Autodesk Inventor part; units mm, degrees
ref_plane "YZ Plane" through (0, 0, 0) normal (1, 0, 0) x (0, 1, 0)
ref_plane "XZ Plane" through (0, 0, 0) normal (0, 1, 0) x (-1, 0, 0)
ref_plane "XY Plane" through (0, 0, 0) normal (0, 0, 1) x (1, 0, 0)
sketch "Sketch1" plane through (0, 0, 0) normal (0, 0, 1) x (1, 0, 0)
  line L0 (10.3923, 0) -> (5.1962, -9)
  line L1 (5.1962, -9) -> (-5.1962, -9)
  line L2 (-5.1962, -9) -> (-10.3923, 0)
  line L3 (-10.3923, 0) -> (-5.1962, 9)
  line L4 (-5.1962, 9) -> (5.1962, 9)
  line L5 (5.1962, 9) -> (10.3923, 0)
  point P0 (0, 0)
  point P1 (0, 0)
  dimension "d0" = 18
extrude "Extrusion1" add sketch "Sketch1" along normal blind 2.8
sketch "Sketch2" plane through (0, 0, 2.8) normal (0, 0, 1) x (1, 0, 0)
  circle A0 centre (0, 0) radius 6
  dimension "d3" = 12
extrude "Extrusion2" cut sketch "Sketch2" against normal through all
chamfer "Chamfer1" distance 1 angle 45 6 edges at (5.1962, 9, 1.4) (-5.1962, 9, 1.4) (10.3923, 0, 1.4) (5.1962, -9, 1.4) (-5.1962, -9, 1.4) (-10.3923, 0, 1.4)
chamfer "Chamfer2" distance 0.5 angle 45 12 edges at (-9.8923, 0, 2.8) (-4.9462, -8.567, 2.8) (4.9462, -8.567, 2.8) (9.8923, 0, 2.8) (4.9462, 8.567, 2.8) (-4.9462, 8.567, 2.8) (-4.9462, 8.567, 0) (-9.8923, 0, 0) (-4.9462, -8.567, 0) (4.9462, -8.567, 0) (9.8923, 0, 0) (4.9462, 8.567, 0)
properties part number "c-t4140012051-000-a-3d_NUT"
Verification items for the finished model (mm, model axes). Coordinates: 2 decimals unless noted, no trailing zeros. Write each loop counter-clockwise with the first axis right and the second up, starting at its lowest first coordinate (ties: lowest second). Pieces come first, ordered by that corner, then holes. Notation, with made-up numbers: M 52,46 L 59,46 A23 ccw 59,59 Z; hole C 7.25,-35.5 d8. An arc over 180 degrees is marked long. Answer as a JSON object with one key per item and string values. Group by question number.
(1) Cross-section at B-B, the plane x = 0. Record the cut outline in (y, z), and give its area (3 significant figures).
(2) Material ranges on line 1 (Y direction, x = 0, z = 1.6); line 2 (X direction, y = -3, z = 2.25); line 3 (X direction, y = 4.25, z = 1.85), recorded low to high.
(3) Cross-section at D-D, the plane y = 3. Record the cut outline in (x, z), and give its area (3 significant figures).
(4) Cross-section at A-A, the plane y = 0. Record the cut outline in (x, z).
(5) Release check for a two-part mould opening along Y. For faces 1 (the face through (-4.77, -8.32, 0.2)), 2 (the face through (-6, 0, 1)), 3 (the face through (4.816, 8.293, 0.198)) record: +Y half, -Y half, draft (parallel to the pull), parting line (faces both ways), or undercut.
(6) Cross-section at C-C, the plane z = 0.25. Record the cut outline in (x, y).
Reply:
{
 "1": {"outline": "M -9,0 L -6,0 L -6,2.8 L -9,2.8 Z; M 6,0 L 9,0 L 9,2.8 L 6,2.8 Z", "area": "16.8 mm²"},
 "2": {"line 1": "-9 to -6, 6 to 9", "line 2": "-8.66 to -5.2, 5.2 to 8.66", "line 3": "-7.94 to -4.24, 4.24 to 7.94"},
 "3": {"outline": "M -8.66,0 L -5.2,0 L -5.2,2.8 L -8.66,2.8 Z; M 5.2,0 L 8.66,0 L 8.66,2.8 L 5.2,2.8 Z", "area": "19.4 mm²"},
 "4": {"outline": "M -9.89,0.5 L -9.39,0 L -6,0 L -6,2.8 L -9.39,2.8 L -9.89,2.3 Z; M 6,0 L 9.39,0 L 9.89,0.5 L 9.89,2.3 L 9.39,2.8 L 6,2.8 Z"},
 "5": {"face 1": "-Y half", "face 2": "undercut", "face 3": "+Y half"},
 "6": {"outline": "M -9.64,-1.3 L -5.95,-7.7 L -3.7,-9 L 3.7,-9 L 5.95,-7.7 L 9.64,-1.3 L 9.64,1.3 L 5.95,7.7 L 3.7,9 L -3.7,9 L -5.95,7.7 L -9.64,1.3 Z; hole C 0,0 d12"}
}
